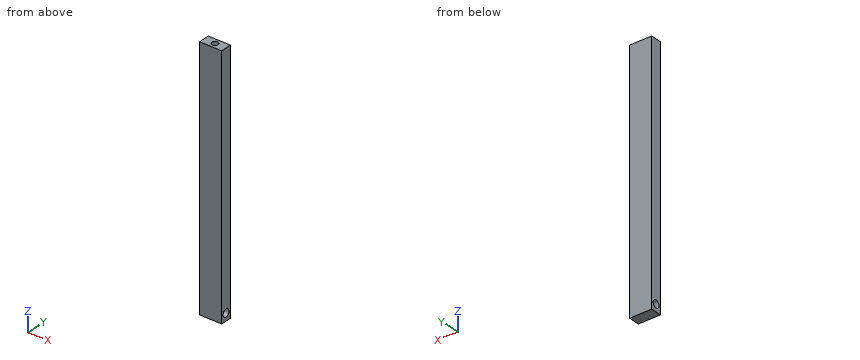
```python
from build123d import *

# Parameters (mm, degrees)
F0_W     = 38.1
F0_H     = 431.8
F1_DEPTH = 9.525
F3_D     = 12.7
F5_D     = 10.71626
F5_DEPTH = 38.0941384615
F5_TIP   = 3.2194893086


# Not quite as in the source:
# - a length typed as a fraction of an inch, garbled in the dataset ("3 / 203.2 mm" for 3/8 in), is restored


with BuildPart() as f1:
    # F0 (on Front) → F1 (new body, symmetric)
    with BuildSketch(Plane.XZ):
        Rectangle(F0_W, F0_H)
    extrude(amount=F1_DEPTH, both=True)

    # F3 (through all)
    with Locations(Plane.YZ.offset(19.05)):
        with Locations((0, -203.2)):
            Hole(F3_D / 2)

    # F5
    with Locations(Plane.XY.offset(215.9)):
        with Locations((0, 0)):
            Hole(F5_D / 2, depth=F5_DEPTH)
            with Locations((0, 0, -(F5_DEPTH + F5_TIP / 2))):  # 118° drill point
                Cone(0, F5_D / 2, F5_TIP, mode=Mode.SUBTRACT)


solid = f1.part
```
Read the model definition and answer for the solid it produces. Units are mm, in the model's axes. Give positions to 0.01 mm unless a question says otherwise; leave off trailing zeros. Loops run counter-clockwise (first coordinate to the right, second up) from the corner with the lowest first, then second, coordinate; pieces in that order, holes last.
Item 1: Find the intervals of material crossed by line 1 along Z through (x, y) = (6, 0.5); line 2 along X through (y, z) = (0, 208); line 3 along Y through (x, z) = (8, -203) (3 decimals), in increasing order.
Item 2: The part is cut by section A-A (z = -203.2). Write down the section's boundary in (x, y) (3 decimals).
Item 3: Each of these flat-tipped pins is pushed along its axis until it touches: pin 1 Ø1.5 at (x, y) = (0.5, 4) entering from +Z; pin 2 Ø8.5 at (x, y) = (0, 0) entering from +Z. Where does it stop, or does it pass through?
Taken from the geometry:
1. line 1: z = -215.9 to -209.53, -196.87 to 215.9
1. line 2: x = -19.05 to -5.36, 5.36 to 19.05
1. line 3: y = -9.525 to -6.347, 6.347 to 9.525
2. outline: (-19.05, -9.525) - (19.05, -9.525) - (19.05, -6.35) - (-19.05, -6.35) - close; (-19.05, 6.35) - (19.05, 6.35) - (19.05, 9.525) - (-19.05, 9.525) - close
3. pin 1: stops at z = 177.46
3. pin 2: stops at z = 177.14
